Autodesk Inventor part; units mm, degrees
ref_plane "YZ Plane" through (0, 0, 0) normal (1, 0, 0) x (0, 1, 0)
ref_plane "XZ Plane" through (0, 0, 0) normal (0, 1, 0) x (-1, 0, 0)
ref_plane "XY Plane" through (0, 0, 0) normal (0, 0, 1) x (1, 0, 0)
sketch "Szkic1" plane through (0, 0, 0) normal (0, 0, 1) x (1, 0, 0)
  arc A0 (-0.9737, -7.4365) -> (-5.9534, -4.5615) centre (0, 0) ccw
  circle A1 centre (0, 0) radius 4
  circle A2 centre (0, -5.75) radius 0.5
  circle A3 centre (3.1597, -4.8041) radius 0.5
  circle A4 centre (5.2797, -2.2775) radius 0.5
  circle A5 centre (5.6626, 0.9985) radius 0.5
  circle A6 centre (4.1824, 3.9459) radius 0.5
  circle A7 centre (1.326, 5.595) radius 0.5
  circle A8 centre (-1.9666, 5.4032) radius 0.5
  circle A9 centre (-4.6122, 3.4337) radius 0.5
  circle A10 centre (-5.7403, 0.3343) radius 0.5
  circle A11 centre (-4.9796, -2.875) radius 0.5
  arc A12 (-5.4821, -5.4952) -> (-5.9534, -4.5615) centre (-8.3548, -6.3596) ccw
  arc A13 (-0.9737, -7.4365) -> (-2.0179, -7.4952) centre (-1.3301, -10.4153) ccw
  line L0 (-5.4821, -5.4952) -> (-5.9821, -6.3612)
  line L1 (-2.0179, -7.4952) -> (-2.5179, -8.3612)
  line L2 (-2.5179, -8.3612) -> (-5.9821, -6.3612)
  dimension "d0" = 15
  dimension "d1" = 8
  dimension "d2" = 1
  dimension "d5" = 300
extrude "Wyciągnięcie proste1" add sketch "Szkic1" along normal mid plane 0.5
sketch "Szkic2" plane through (0, 0, 0.25) normal (0, 0, 1) x (1, 0, 0)
  line L0 (-5.9821, -6.3612) -> (-2.5179, -8.3612)
  line L1 (-2.2679, -7.9282) -> (-5.7321, -5.9282)
  line L2 (-5.7321, -5.9282) -> (-5.9821, -6.3612)
  line L3 (-2.2679, -7.9282) -> (-2.5179, -8.3612)
extrude "Wyciągnięcie proste2" add sketch "Szkic2" along normal blind 1
fillet "Zaokrąglenie1" radius 0.5 1 edges at (-4.25, -7.3612, -0.25)
fillet "Zaokrąglenie2" radius 0.25 1 edges at (-4, -6.9282, 0.25)
properties part number "SŁONECZKO MAŁE Z BLOKADĄ" material "Stal"
Part model, mm, in its own coordinate system. Coordinates: 2 decimals unless noted, no trailing zeros. Order: outer loops, then holes, each group sorted by start corner. A loop starts at its lowest first (then second) coordinate and runs counter-clockwise, first axis right, second up. Notation, with made-up numbers: (-3, -25) -> (27, -25) arc R21 ccw to (27, -13) -> close; hole circle Ø3 at (-36.5, -0.75). An arc over 180 degrees is marked (long way). Put each result on its own line as item: value. Start each with the question number.
(1) Probe line 1 along Y through (x, z) = (0, 0.1); line 2 along X through (y, z) = (1.75, 0.1); line 3 along Z through (x, y) = (2.5, 6.5). List the from-to ranges inside material, lowest first. Write a range as [from, to].
(2) Band-saw the part on C-C (y = 2.5). Give the cut face in (x, z).
(3) Mould opens along Y. For faces 1 (the face through (-5.84, -6.115, 0.323)), 2 (the face through (3, -3, 0.25)), 3 (the face through (-4.199, -7.217, -0.107)), 4 (the face through (4.78, -2.3, 0)) say: pulls with the +Y half, pulls with the -Y half, needs draft (parallel to the pull), parting line crosses it, or undercut.
(4) Pin check, flat tip, straight feed: pin 1 Ø1 at (x, y) = (-0.5, -5) entering from +Z. Stop position of the tip, or through.
(5) Band-saw the part on B-B (y = -2). Give the cut face in (x, z).
(6) Band-saw the part on D-D (z = 0.95). Give the cut face in (x, y), then the cut area to 3 significant figures.
(7) Band-saw the part on A-A (x = 0). Give the cut face in (y, z).
Determined:
1. line 1: y = [-7.5, -6.25], [-5.25, -4], [4, 7.5]
1. line 2: x = [-7.29, -3.6], [3.6, 7.29]
1. line 3: z = [-0.25, 0.25]
2. outline: (-7.07, -0.25) -> (-3.12, -0.25) -> (-3.12, 0.25) -> (-7.07, 0.25) -> close; (3.12, -0.25) -> (7.07, -0.25) -> (7.07, 0.25) -> (3.12, 0.25) -> close
3. face 1: undercut
3. face 2: needs draft
3. face 3: pulls with the -Y half
3. face 4: undercut
4. pin 1: stops at z = 0.25
5. outline: (-7.23, -0.25) -> (-3.46, -0.25) -> (-3.46, 0.25) -> (-7.23, 0.25) -> close; (3.46, -0.25) -> (4.86, -0.25) -> (4.86, 0.25) -> (3.46, 0.25) -> close; (5.7, -0.25) -> (7.23, -0.25) -> (7.23, 0.25) -> (5.7, 0.25) -> close
6. outline: (-5.98, -6.36) -> (-2.52, -8.36) -> (-2.27, -7.93) -> (-5.73, -5.93) -> close
6. area: 2.00 mm²
7. outline: (-7.5, -0.25) -> (-6.25, -0.25) -> (-6.25, 0.25) -> (-7.5, 0.25) -> close; (-5.25, -0.25) -> (-4, -0.25) -> (-4, 0.25) -> (-5.25, 0.25) -> close; (4, -0.25) -> (7.5, -0.25) -> (7.5, 0.25) -> (4, 0.25) -> close
